```python
from build123d import *

# Parameters (mm, degrees)
F0_R     = 4.7625
F1_DEPTH = 76.2


# Not quite as in the source:
# - the program builds the solid bodies; features that only make, move or delete a surface that nothing else refers to are left out


with BuildPart() as f1:
    # F0 (on Front) → F1 (new body)
    with BuildSketch(Plane.XZ):
        with BuildLine():
            Line((-114.3, 0), (0, 0))
            Line((0, 0), (0, 19.05))
            Line((0, 19.05), (-114.3, 19.05))
            Line((-114.3, 19.05), (-114.3, 14.2229856587))
            Line((-114.3, 14.2229856587), (-108.7215644084, 14.2229856587))
            ThreePointArc((-108.7215644084, 14.2229856587), (-105.2435953967, 12.891306681), (-103.7874654915, 9.4635781261))
            ThreePointArc((-103.7874654915, 9.4635781261), (-105.1136603504, 6.1661225575), (-108.3536442745, 4.7051262529))
            ThreePointArc((-108.3536442745, 4.7051262529), (-108.5499654915, 4.7010781261), (-108.7462867086, 4.7051262529))
            Line((-108.7462867086, 4.7051262529), (-114.3, 4.7051262529))
            Line((-114.3, 4.7051262529), (-114.3, 0))
        make_face()
        with Locations((-9.4899654915, 9.609828106)):
            Circle(F0_R, mode=Mode.SUBTRACT)
    extrude(amount=F1_DEPTH)


solid = f1.part
```
The listing builds one solid part. Answer for the finished solid, in the listing's coordinates (mm). A direction names the side the tool comes from. Give positions to 0.01 mm unless a question says otherwise; leave off trailing zeros. Use one line per item in the form item = value. Start each with the question number.
1) A tool of negligible diameter and unlimited length cuts with its end or side. For faces 1 (the face through (-58, -76.2, 10)), 2 (the face through (-112, -38, 14.223)), from which of +Z, -Z, +X, -X, +Y, -Y can it reach the whole face along a straight path? Write none if from no direction.
2) The mould has two halves that part along Z. Classify faces 3 (the face through (-58, -38, 0)), 4 (the face through (-111, -38, 4.705)), 5 (the face through (-114.3, -38, 2)): pulls with the +Z half, pulls with the -Z half, needs draft (parallel to the pull), parting line crosses it, or undercut.
3) A flat-ended cylindrical pin translates along its axis: pin 1 Ø10 at (y, z) = (-67.5, 11) entering from +X. Find the tip coordinate at first contact, or state that the pin passes through.
4) Consider line 1 along X through (y, z) = (-60, 5.5); line 2 along X through (y, z) = (-63, 13.5); line 3 along Z through (x, y) = (-105, -57). Determine where each line is inside the solid, lowest interval first. Write a range as from..to.
Geometry results:
q1.face_1 = +Z, -Z, +X, -X, -Y
q1.face_2 = -X, +Y, -Y
q2.face_3 = pulls with the -Z half
q2.face_4 = undercut
q2.face_5 = needs draft
q3.pin_1 = 0
q4.line_1 = -105.91..-11.9, -7.08..0
q4.line_2 = -106.02..-12.24, -6.74..0
q4.line_3 = 0..6.29, 12.64..19.05
